Model file for the job. Use its own axes, mm. A direction names the side the tool comes from. Give positions to 0.01 mm unless a question says otherwise; leave off trailing zeros. Loops run counter-clockwise (first coordinate to the right, second up) from the corner with the lowest first, then second, coordinate; pieces in that order, holes last. Notation, with made-up numbers: M 9,48 L 31,48 A21 ccw 31,59 Z; hole C 9,73.25 d7. An arc over 180 degrees is marked long. Use CSV: the item, a comma, the result in double quotes. Start each with the question number.
(1) Slice it at C-C on y = 8. List the corners of the cut face in (x, z).
(2) Flat gauge pins, fed straight in: P1, Ø4, axis at x = -2, z = -51.5, coming from the -Y side; P2, Ø1.5, axis at x = 3, y = 2, coming from the -Z side. Where does each tip first touch, or does it go through?
(3) Slice it at D-D on y = 0.75. List the corners of the cut face in (x, z).
(4) Two-plate mould, pull along X, no slides. Class faces 3 (the face through (0.32, 6.55, -51.53)), 4 (the face through (5.9, 6.55, -64.43)), 5 (the face through (0, 3, -38)): pulls with the +X half, pulls with the -X half, needs draft (parallel to the pull), parting line crosses it, or undercut.
(5) Tool access for faces 1 (the face through (3.96, 4.93, -0.52)), 2 (the face through (0, 1, -12)): list every direction of +Z, -Z, +X, -X, +Y, -Y with a clear straight run to the whole face (end or side of a thin tool).
(6) Slice it at A-A on x = 0. List the corners of the cut face in (y, z), and give its area (3 significant figures).
(7) Slice it at B-B on z = -54. List the corners of the cut face in (x, y).
(8) Wall check: line 1 along Z through (x, y) = (-0.25, 4.25); line 2 along Z through (x, y) = (-1, 6.25); line 3 along Y through (x, z) = (-5.5, -33.5). Give the ranges that are in metal, low to high. Write a range as from..to.
```python
from build123d import *

# Parameters (mm, degrees)
SKETCH1_R                  = 3.99415
BOSS_EXTRUDE1_DEPTH        = 10
SKETCH2_W                  = 13
SKETCH2_H                  = 53
CUT_EXTRUDE1_DEPTH         = 3
F_10_CLEARANCE_HOLE1_D     = 4.9784
F_10_CLEARANCE_HOLE1_DEPTH = 40
F_10_CLEARANCE_HOLE1_TIP   = 1.495662253
FILLET1_R                  = 2


with BuildPart() as part:
    # Sketch1 → Boss-Extrude1 (new body)
    with BuildSketch(Plane(origin=(0, 0, 0), x_dir=(1, 0, 0), z_dir=(0, 1, 0))):
        with BuildLine():
            Line((-6.5, 0), (-6.5, 65))
            Line((-6.5, 65), (6.5, 65))
            Line((6.5, 65), (6.5, 0))
            ThreePointArc((6.5, 0), (0, -6.5), (-6.5, 0))
        make_face()
        with Locations(Location((0, 0, 0), (0, 0, 270))):  # turned: the seam where the file's is
            Circle(SKETCH1_R, mode=Mode.SUBTRACT)
    extrude(amount=BOSS_EXTRUDE1_DEPTH)

    # Sketch2 → Cut-Extrude1 (cut)
    with BuildSketch(Plane.XZ):
        with Locations((0, -38.5)):
            Rectangle(SKETCH2_W, SKETCH2_H)
    extrude(amount=-CUT_EXTRUDE1_DEPTH, mode=Mode.SUBTRACT)

    # #10 Clearance Hole1
    with Locations(Plane.XZ.offset(-3)):
        with Locations((0, -54), (0, -24)):
            Hole(F_10_CLEARANCE_HOLE1_D / 2, depth=F_10_CLEARANCE_HOLE1_DEPTH)
            with Locations((0, 0, -(F_10_CLEARANCE_HOLE1_DEPTH + F_10_CLEARANCE_HOLE1_TIP / 2))):  # 118° drill point
                Cone(0, F_10_CLEARANCE_HOLE1_D / 2, F_10_CLEARANCE_HOLE1_TIP, mode=Mode.SUBTRACT)

    # Fillet1
    fillet1_edges = [part.edges().sort_by_distance(p)[0] for p in [
        (-6.5, 6.5, -65),
        (6.5, 6.5, -65),
    ]]
    fillet(fillet1_edges, radius=FILLET1_R)


solid = part.part
```
Reply:
1,outline,"M -6.5,-63 A2 ccw -4.5,-65 L 4.5,-65 A2 ccw 6.5,-63 L 6.5,0 A6.5 ccw -6.5,0 Z; hole C 0,0 d7.99; hole C 0,-54 d4.98; hole C 0,-24 d4.98"
2,P1,"stops at y = 3"
2,P2,"stops at z = -12"
3,outline,"M -6.5,-12 L 6.5,-12 L 6.5,0 A6.5 ccw -6.5,0 Z; hole C 0,0 d7.99"
4,face 3,"undercut"
4,face 4,"pulls with the +X half"
4,face 5,"needs draft"
5,face 1,"+Y, -Y"
5,face 2,"-Z, +X, -X, -Y"
6,outline,"M 0,-12 L 3,-12 L 3,-21.51 L 10,-21.51 L 10,-3.99 L 0,-3.99 Z; M 0,3.99 L 10,3.99 L 10,6.5 L 0,6.5 Z; M 3,-65 L 10,-65 L 10,-56.49 L 3,-56.49 Z; M 3,-51.51 L 10,-51.51 L 10,-26.49 L 3,-26.49 Z"
6,area,"406 mm^2"
7,outline,"M -6.5,3 L -2.49,3 L -2.49,10 L -6.5,10 Z; M 2.49,3 L 6.5,3 L 6.5,10 L 2.49,10 Z"
8,line 1,"z = -65..-56.48, -51.52..-26.48, -21.52..-3.99, 3.99..6.5"
8,line 2,"z = -65..-56.28, -51.72..-26.28, -21.72..-3.87, 3.87..6.42"
8,line 3,"y = 3..10"
